Build history of the part. All positions in model axes, mm. Face numbers are marked on the shaded views. A direction names the side the tool comes from. Round coordinates to 2 decimals unless told otherwise and drop trailing zeros. Write each loop counter-clockwise with the first axis right and the second up, starting at its lowest first coordinate (ties: lowest second). Pieces come first, ordered by that corner, then holes.
Item 1: Band-saw the part on A-A, the plane y = 9.25. Write the cut outline in (x, z).
Item 2: Band-saw the part on D-D, the plane y = 18. Write the cut outline in (x, z), then the cut area to 3 significant figures.
Item 3: Band-saw the part on C-C, the plane z = -13. Write the cut outline in (x, y), then the cut area to 3 significant figures.
Item 4: Mould opens along X. For the marked faces 1, 2, 3 and 4 say: +X half, -X half, draft (parallel to the pull), parting line (faces both ways), or undercut.
Item 5: Band-saw the part on B-B, the plane x = 13.75. Write the cut outline in (y, z).
Item 6: Drop flat-ended pins along their axis: pin 1 Ø14 at (x, y) = (6.5, 17) entering from +Z; pin 2 Ø3.5 at (y, z) = (2, -3) entering from +X; pin 3 Ø3 at (x, z) = (-5, -5) entering from +Y; pin 4 Ø0.9 at (y, z) = (2, -5) entering from -X. Give the stop position or say it passes through.
Item 7: 3-axis set-ups, long thin cutter, end or side, ignore diameter. For the marked faces 5, 6 and 7: which of +Z, -Z, +X, -X, +Y, -Y reach the whole face in a straight line?
Item 8: Wall check: probe 1 along X at (y, z) = (18, -19); probe 2 along Y at (x, z) = (13.75, -23); probe 3 along X at (y, z) = (24, -25.5). Give the ranges that are in metal, low to high.
Autodesk Inventor part; units mm, degrees
ref_plane "YZ Plane" through (0, 0, 0) normal (1, 0, 0) x (0, 1, 0)
ref_plane "XZ Plane" through (0, 0, 0) normal (0, 1, 0) x (-1, 0, 0)
ref_plane "XY Plane" through (0, 0, 0) normal (0, 0, 1) x (1, 0, 0)
sketch "Sketch1" plane through (0, 0, 0) normal (0, 1, 0) x (-1, 0, 0)
  line L0 (0, 0) -> (10, 0)
  line L1 (10, 0) -> (10, -27)
  line L2 (10, -27) -> (0, -27)
  line L3 (0, -27) -> (0, 0)
  dimension "d0" = 10
  dimension "d1" = 27
extrude "Extrusion1" add sketch "Sketch1" along normal blind 10
sketch "Sketch2" plane through (0, 10, 0) normal (0, 1, 0) x (1, 0, 0)
  line L0 (-10, 27) -> (-10, 0)
  line L1 (-10, 0) -> (-10, 5)
  circle A0 centre (-5, 5) radius 2.55
  point P0 (0, 0)
  dimension "d4" = 5
  dimension "d5" = 5.1
extrude "Extrusion2" cut sketch "Sketch2" against normal blind 10
sketch "Sketch4" plane through (0, 10, 0) normal (0, 1, 0) x (1, 0, 0)
  line L0 (0, 27) -> (-10, 27)
  line L1 (-10, 27) -> (-10, 0)
  line L2 (0, 27) -> (-10, 27)
  line L3 (-10, 27) -> (-10, 0)
  line L4 (-10, 0) -> (0, 0)
  line L5 (0, 0) -> (0, 27)
  point P0 (0, 0)
  dimension "d13" = 27
extrude "Extrusion4" cut sketch "Sketch4" against normal blind 7
sketch "Sketch5" plane through (0, 3, 0) normal (0, 1, 0) x (1, 0, 0)
  line L0 (-10, 27) -> (0, 27)
  line L1 (-5, 27) -> (17.5, 27)
  line L2 (17.5, 27) -> (17.5, 12)
  line L3 (17.5, 12) -> (-5, 12)
  line L4 (-5, 12) -> (-5, 27)
  line L5 (-5, 27) -> (-27.5, 27)
  line L6 (-27.5, 27) -> (-27.5, 12)
  line L7 (-27.5, 12) -> (-5, 12)
  line L8 (-5, 12) -> (-5, 27)
  point P0 (0, 0)
  dimension "d16" = 22.5
  dimension "d17" = 15
  dimension "d18" = 22.5
extrude "Extrusion5" add sketch "Sketch5" against normal blind 3
sketch "Sketch6" plane through (0, 3, 0) normal (0, 1, 0) x (1, 0, 0)
  line L0 (17.5, 12) -> (-27.5, 12)
  line L1 (-5, 12) -> (10, 12)
  line L2 (10, 12) -> (10, 27)
  line L3 (-27.5, 27) -> (17.5, 27)
  line L4 (-5, 12) -> (-20, 12)
  line L5 (-27.5, 12) -> (-10, 12)
  line L6 (-20, 12) -> (-20, 27)
  line L7 (-20, 12) -> (-27.5, 12)
  line L8 (-27.5, 12) -> (-27.5, 27)
  line L9 (-27.5, 27) -> (-20, 27)
  line L10 (-20, 27) -> (-20, 12)
  line L11 (10, 12) -> (17.5, 12)
  line L12 (17.5, 12) -> (17.5, 27)
  line L13 (17.5, 27) -> (10, 27)
  line L14 (10, 27) -> (10, 12)
  point P0 (0, 0)
  dimension "d21" = 15
  dimension "d22" = 15
extrude "Extrusion6" add sketch "Sketch6" along normal blind 25 contours L0 L2 L3 L12 | L6 L0 L8 L3
sketch "Sketch7" plane through (17.5, 0, -27) normal (0, 0, -1) x (-1, 0, 0)
  line L0 (37.5, 3) -> (7.5, 3)
  line L1 (7.5, 3) -> (0, 3)
  line L2 (0, 0) -> (0, 28)
  line L3 (3.75, 3) -> (3.75, 18)
  line L4 (37.5, 3) -> (44.9906, 3)
  line L5 (41.2453, 3) -> (41.2453, 18)
  circle A0 centre (3.75, 18) radius 1.75
  circle A1 centre (41.2453, 18) radius 1.75
  point P0 (17.5, 0)
  dimension "d25" = 15
  dimension "d26" = 15
  dimension "d27" = 3.5
  dimension "d28" = 3.5
extrude "Extrusion7" cut sketch "Sketch7" against normal blind 25
properties part number "Raket_Arme_Motor"
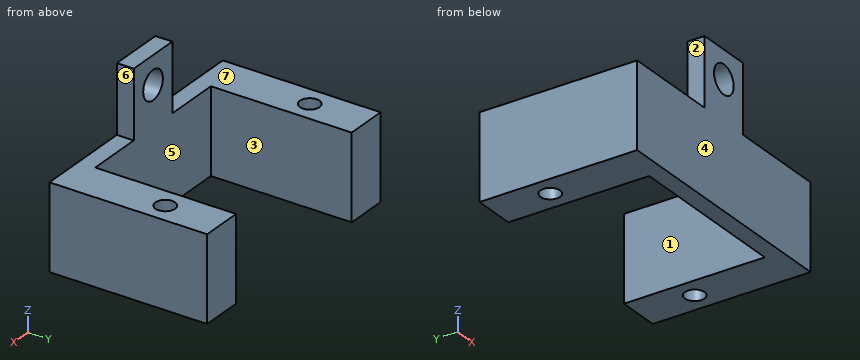
Results:
1. outline: (-27.5, -27) - (-20, -27) - (-20, -12) - (-27.5, -12) - close; (10, -27) - (17.5, -27) - (17.5, -12) - (10, -12) - close
2. outline: (-27.5, -27) - (-25.5, -27) - (-25.5, -12) - (-27.5, -12) - close; (-22, -27) - (-20, -27) - (-20, -12) - (-22, -12) - close; (10, -27) - (12, -27) - (12, -12) - (10, -12) - close; (15.5, -27) - (17.5, -27) - (17.5, -12) - (15.5, -12) - close
2. area: 120 mm2
3. outline: (-27.5, 0) - (17.5, 0) - (17.5, 28) - (10, 28) - (10, 3) - (-20, 3) - (-20, 28) - (-27.5, 28) - close; hole circle Ø3.5 at (-23.75, 18); hole circle Ø3.5 at (13.75, 18)
3. area: 491 mm2
4. face 1: undercut
4. face 2: -X half
4. face 3: undercut
4. face 4: draft
5. outline: (0, -27) - (16.25, -27) - (16.25, -12) - (0, -12) - close; (19.75, -27) - (28, -27) - (28, -12) - (19.75, -12) - close
6. pin 1: stops at z = -12
6. pin 2: stops at x = 0
6. pin 3: passes through
6. pin 4: stops at x = -10
7. face 5: +Z, -Z, +Y
7. face 6: +Z, +X, +Y, -Y
7. face 7: +Z, -X, +Y, -Y
8. probe 1: x = -27.5 to -25.5, -22 to -20, 10 to 12, 15.5 to 17.5
8. probe 2: y = 0 to 16.25, 19.75 to 28
8. probe 3: x = -27.5 to -20, 10 to 17.5
